from build123d import *

# Parameters (mm, degrees)
SALIENTE_EXTRUIR1_DEPTH = 12.5
CROQUIS2_R              = 8.5
CORTAR_EXTRUIR1_DEPTH   = 41.25
CROQUIS3_R              = 8.5
CORTAR_EXTRUIR2_DEPTH   = 82.5
CROQUIS4_R              = 1.5875
CORTAR_EXTRUIR3_DEPTH   = 82.5


with BuildPart() as part:
    # Croquis1 → Saliente-Extruir1 (new body)
    with BuildSketch(Plane.XY):
        with BuildLine():
            Line((-20, -30), (20, -30))
            ThreePointArc((20, -30), (27.071067812, -27.071067812), (30, -20))
            Line((30, -20), (30, 20))
            ThreePointArc((30, 20), (27.071067812, 27.071067812), (20, 30))
            Line((20, 30), (-20, 30))
            ThreePointArc((-20, 30), (-27.071067812, 27.071067812), (-30, 20))
            Line((-30, 20), (-30, -20))
            ThreePointArc((-30, -20), (-27.071067812, -27.071067812), (-20, -30))
        make_face()
    extrude(amount=SALIENTE_EXTRUIR1_DEPTH)

    # Croquis2 → Cortar-Extruir1 (cut, symmetric)
    with BuildSketch(Plane(origin=(0, 0, 0), x_dir=(1, 0, 0), z_dir=(0, 1, 0))):
        Circle(CROQUIS2_R)
    extrude(amount=CORTAR_EXTRUIR1_DEPTH, both=True, mode=Mode.SUBTRACT)

    # Croquis3 → Cortar-Extruir2 (cut)
    with BuildSketch(Plane.ZY.offset(30)):
        Circle(CROQUIS3_R)
    extrude(amount=-CORTAR_EXTRUIR2_DEPTH, mode=Mode.SUBTRACT)

    # Croquis4 → Cortar-Extruir3 (cut)
    with BuildSketch(Plane.XY.offset(12.5)):
        with Locations((-20, 20)):
            Circle(CROQUIS4_R)
        with Locations((20, 20)):
            Circle(CROQUIS4_R)
        with Locations((20, -20)):
            Circle(CROQUIS4_R)
        with Locations((-20, -20)):
            Circle(CROQUIS4_R)
    extrude(amount=-CORTAR_EXTRUIR3_DEPTH, mode=Mode.SUBTRACT)


solid = part.part
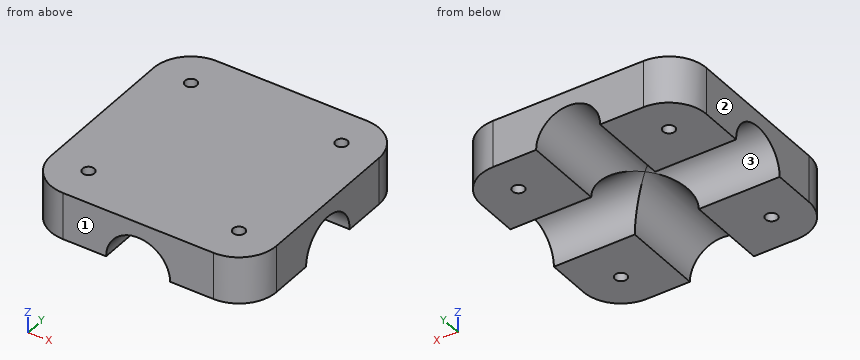
Input: part model. Units: mm. Frame: model coordinates. Face numbers are marked on the shaded views. Give positions to 0.01 mm unless a question says otherwise; leave off trailing zeros. Loops run counter-clockwise (first coordinate to the right, second up) from the corner with the lowest first, then second, coordinate; pieces in that order, holes last. Notation, with made-up numbers: M 85,-19 L 120,-19 A22 ccw 120,-13 Z; hole C 60,-5 d5. An arc over 180 degrees is marked long. Use one line per item in the form item = value.
1. Pull-direction query (Y, two-part tool) for the marked faces 1, 2 and 3; classes: released by +Y, released by -Y, zero draft, split by the parting line, or undercut.
Numbers:
face_1 = released by -Y
face_2 = zero draft
face_3 = undercut
2. Section query C-C, the plane x = 10. Return the cut outline in (y, z).
Numbers:
outline = M -30,0 L -8.5,0 A8.5 cw 8.5,0 L 30,0 L 30,12.5 L -30,12.5 Z
3. Section query B-B, the plane y = -26. Return the cut outline in (x, z).
Numbers:
outline = M -28,0 L -8.5,0 A8.5 cw 8.5,0 L 28,0 L 28,12.5 L -28,12.5 Z
4. Line query: L1, parallel to Y at x = -20, z = 9.25; L2, parallel to Y at x = -15.5, z = 0.5. Output: solid intervals per line, ascending.
Numbers:
L1 = -30 to -21.59, -18.41 to 18.41, 21.59 to 30
L2 = -30 to -8.49, 8.49 to 30
5. Section query A-A, the plane z = 4. Return the cut outline in (x, y) (1 decimal).
Numbers:
outline = M -30,-20 A10 ccw -20,-30 L -7.5,-30 L -7.5,-7.5 L -30,-7.5 Z; M -30,7.5 L -7.5,7.5 L -7.5,30 L -20,30 A10 ccw -30,20 Z; M 7.5,-30 L 20,-30 A10 ccw 30,-20 L 30,-7.5 L 7.5,-7.5 Z; M 7.5,7.5 L 30,7.5 L 30,20 A10 ccw 20,30 L 7.5,30 Z; hole C -20,-20 d3.2; hole C -20,20 d3.2; hole C 20,-20 d3.2; hole C 20,20 d3.2
6. Section query D-D, the plane z = 7.75. Return the cut outline in (x, y) (1 decimal).
Numbers:
outline = M -30,-20 A10 ccw -20,-30 L -3.5,-30 L -3.5,-3.5 L -30,-3.5 Z; M -30,3.5 L -3.5,3.5 L -3.5,30 L -20,30 A10 ccw -30,20 Z; M 3.5,-30 L 20,-30 A10 ccw 30,-20 L 30,-3.5 L 3.5,-3.5 Z; M 3.5,3.5 L 30,3.5 L 30,20 A10 ccw 20,30 L 3.5,30 Z; hole C -20,-20 d3.2; hole C -20,20 d3.2; hole C 20,-20 d3.2; hole C 20,20 d3.2
7. First-contact query: pin 1 (3 mm diameter, centred on x = -1, y = -23.5, fed in from -Z); pin 2 (2 mm diameter, centred on x = 20.5, y = 0, fed in from -Z). Flat tips, straight axial feed; report the tip coordinate or a pass-through.
Numbers:
pin_1 = 8.12
pin_2 = 8.44
